Verification items for the finished model (mm, model axes). Give positions to 0.01 mm unless a question says otherwise; leave off trailing zeros. Loops run counter-clockwise (first coordinate to the right, second up) from the corner with the lowest first, then second, coordinate; pieces in that order, holes last. Notation, with made-up numbers: M 17.5,84.25 L 21.5,84.25 A24 cw 21.5,112.25 Z; hole C -3.75,41.25 d2. An arc over 180 degrees is marked long. Use CSV: the item, a comma, the result in double quotes.
Autodesk Inventor part; units mm, degrees
ref_plane "YZ Plane" through (0, 0, 0) normal (1, 0, 0) x (0, 1, 0)
ref_plane "XZ Plane" through (0, 0, 0) normal (0, 1, 0) x (-1, 0, 0)
ref_plane "XY Plane" through (0, 0, 0) normal (0, 0, 1) x (1, 0, 0)
sketch "Sketch1" plane through (0, 0, 0) normal (0, 1, 0) x (-1, 0, 0)
  line L0 (0, 0) -> (0, -347.765) construction
  line L1 (-3, 0) -> (-3, -347.765)
  line L2 (3, -347.765) -> (3, 0)
  arc A0 (3, 0) -> (-3, 0) centre (0, 0) ccw
  arc A1 (-3, -347.765) -> (3, -347.765) centre (0, -347.765) ccw
  circle A2 centre (0, 0) radius 1.5
  circle A3 centre (0, -347.765) radius 1.5
  circle A4 centre (0, -131.233) radius 1.5
  circle A5 centre (0, -37.934) radius 1.5
  point P0 (0, -173.8825)
  dimension "d0" = 347.765
  dimension "d1" = 6
  dimension "d2" = 3
  dimension "d3" = 3
  dimension "d6" = 3
  dimension "d7" = 131.233
  dimension "d8" = 3
  dimension "d9" = 37.934
extrude "Extrusion1" add sketch "Sketch1" along normal blind 8
sketch "Sketch2" plane through (0, 8, 0) normal (0, 1, 0) x (1, 0, 0)
  arc A0 (3, 347.765) -> (-3, 347.765) centre (0, 347.765) ccw
  line L0 (-3, 347.765) -> (-3, 0)
  arc A1 (-3, 0) -> (3, 0) centre (0, 0) ccw
  line L1 (3, 0) -> (3, 347.765)
  circle A2 centre (0, 131.233) radius 1.5
  circle A3 centre (0, 37.934) radius 1.5
  circle A4 centre (0, 347.765) radius 1.5
  circle A5 centre (0, 0) radius 1.5
(1) Section check B-B on y = 6.5. Record the cut outline in (x, z) (3 decimals), plus the area to 3 significant figures.
Calculated:
outline,"M -3,-347.765 A3 ccw 3,-347.765 L 3,0 A3 ccw -3,0 Z; hole C 0,-347.765 d3; hole C 0,-131.233 d3; hole C 0,-37.934 d3; hole C 0,0 d3"
area,"2,090 mm²"
(2) Depth check by flat-ended pin: pin 1 Ø2.5 at (x, z) = (0, -131.233) entering from -Y; pin 2 Ø1 at (x, y) = (-1, 5.5) entering from +Z. Enter the tip coordinate at first touch or a pass-through.
Calculated:
pin 1,"passes through"
pin 2,"stops at z = 2.96"
(3) Section check A-A on x = 0. Record the cut outline in (y, z) (3 decimals), plus the area to 3 significant figures.
Calculated:
outline,"M 0,-350.765 L 8,-350.765 L 8,-349.265 L 0,-349.265 Z; M 0,-346.265 L 8,-346.265 L 8,-132.733 L 0,-132.733 Z; M 0,-129.733 L 8,-129.733 L 8,-39.434 L 0,-39.434 Z; M 0,-36.434 L 8,-36.434 L 8,-1.5 L 0,-1.5 Z; M 0,1.5 L 8,1.5 L 8,3 L 0,3 Z"
area,"2,730 mm²"
(4) Scan lines: L1, parallel to Z at x = 0, y = 4.5 (3 decimals); L2, parallel to Z at x = -1, y = 2; L3, parallel to Z at x = -2.55, y = 1. Record each from-to range of solid material in increasing order. Write a range as from..to.
Calculated:
L1,"z = -350.765..-349.265, -346.265..-132.733, -129.733..-39.434, -36.434..-1.5, 1.5..3"
L2,"z = -350.59..-348.88, -346.65..-132.35, -130.11..-39.05, -36.82..-1.12, 1.12..2.83"
L3,"z = -349.35..1.58"
